Can you work these out from the drawing? Everything is in mm from the part's minimum corner. Round coordinates to 2 decimals unless told otherwise and drop trailing zeros. Loops run counter-clockwise (first coordinate to the right, second up) from the corner with the lowest first, then second, coordinate; pieces in that order, holes last. Notation, with made-up numbers: (18, -36.75) - (62, -36.75) arc R18 ccw to (62, -19.75) - close; hole circle Ø6 at (57, 50). An arc over 180 degrees is marked (long way). Return JSON: item names as keys, results as strings. Group by question number.
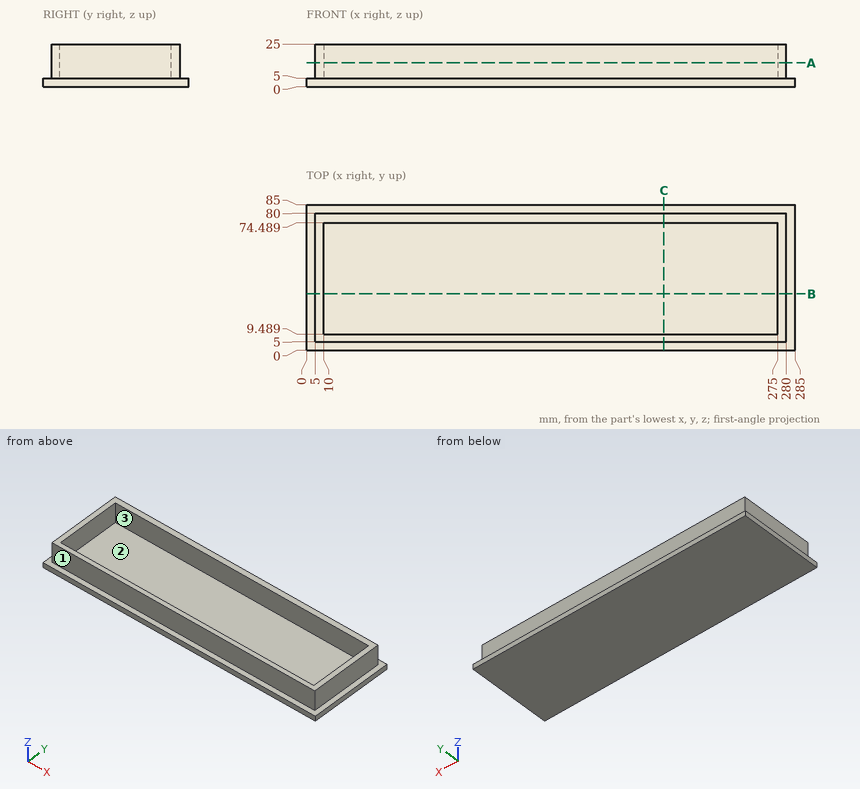
Q1. Imagine slicing it at C-C, the plane x = 208.5. List the corners of the cut face in (y, z) for me.
Q2. Imagine slicing it at A-A, the plane z = 14. List the corners of the cut face in (x, y) for me.
Q3. Will these pins go through, and if not, where does the flat tip stop? pin 1 Ø6 at (x, z) = (159, 16) entering from +Y; pin 2 Ø10 at (x, z) = (89.5, 20) entering from -Y; pin 3 Ø4 at (y, z) = (10.5, 14) entering from -X.
Q4. If we mould it in two halves opening along X, with no side actions, what happens to the marked faces 1, 2 and 3? For each: +X half, -X half, draft (parallel to the pull), parting line (faces both ways), or undercut.
Q5. Please list where these lines run through material, in increasing order: line 1 (Y direction, x = 96, z = 20.5); line 2 (X direction, y = 69, z = 21.5); line 3 (Z direction, x = 206, y = 71).
Q6. Imagine slicing it at B-B, the plane y = 33. List the corners of the cut face in (x, z) for me.
Output values:
{
 "1": {"outline": "(0, 0) - (85, 0) - (85, 5) - (80, 5) - (80, 25) - (74.49, 25) - (74.49, 5) - (9.49, 5) - (9.49, 25) - (5, 25) - (5, 5) - (0, 5) - close"},
 "2": {"outline": "(5, 5) - (280, 5) - (280, 80) - (5, 80) - close; hole (10, 9.49) - (275, 9.49) - (275, 74.49) - (10, 74.49) - close"},
 "3": {"pin 1": "stops at y = 80", "pin 2": "stops at y = 5", "pin 3": "stops at x = 5"},
 "4": {"face 1": "draft", "face 2": "undercut", "face 3": "undercut"},
 "5": {"line 1": "y = 5 to 9.49, 74.49 to 80", "line 2": "x = 5 to 10, 275 to 280", "line 3": "z = 0 to 5"},
 "6": {"outline": "(0, 0) - (285, 0) - (285, 5) - (280, 5) - (280, 25) - (275, 25) - (275, 5) - (10, 5) - (10, 25) - (5, 25) - (5, 5) - (0, 5) - close"}
}
